```python
from build123d import *

# Parameters (mm, degrees)
SKETCH1_R                  = 2.25
BOSS_EXTRUDE1_DEPTH        = 5
M3_5_CLEARANCE_HOLE1_D     = 3.9
M3_5_CLEARANCE_HOLE1_DEPTH = 10
M3_5_CLEARANCE_HOLE1_TIP   = 1.171678207
EXTRUDE_START              = 3
SKETCH_2_R                 = 5
SKETCH_2_R_2               = 1.95
EXTRUDE_2_DEPTH            = 3


with BuildPart() as part:
    # Sketch1 → Boss-Extrude1 (new body)
    with BuildSketch(Plane.XY):
        with BuildLine():
            Line((41.849999868, 40.621529794), (20.610605728, 84.460506241))
            ThreePointArc((20.610605728, 84.460506241), (18.105708126, 87.253517924), (14.499999983, 88.289999977))
            Line((14.499999983, 88.289999977), (-24.945583467, 79.961565754))
            ThreePointArc((-24.945583467, 79.961565754), (-40.125494586, 68.851065128), (-41.843761596, 50.118193373))
            Line((-41.843761596, 50.118193373), (-27.999999977, 9.999999991))
            Line((-27.999999977, 9.999999991), (-22.999999995, 9.999999991))
            Line((-22.999999995, 9.999999991), (-22.999999995, 3.999999991))
            Line((-22.999999995, 3.999999991), (22.999999995, 3.999999991))
            Line((22.999999995, 3.999999991), (22.999999995, 9.999999991))
            Line((22.999999995, 9.999999991), (27.999999977, 9.999999991))
            Line((27.999999977, 9.999999991), (41.849999868, 21.621529803))
            Line((41.849999868, 21.621529803), (41.849999868, 40.621529794))
        make_face()
        with Locations((-29.082392063, 69.767309235)):
            Circle(SKETCH1_R, mode=Mode.SUBTRACT)
        with Locations((-34.70344114, 61.739619201)):
            Circle(SKETCH1_R, mode=Mode.SUBTRACT)
        with Locations(Location((5.43500903, 33.63437382, 0), (0, 0, 180))):
            Circle(SKETCH1_R, mode=Mode.SUBTRACT)
        with Locations(Location((11.056058107, 41.662063854, 0), (0, 0, 180))):
            Circle(SKETCH1_R, mode=Mode.SUBTRACT)
        Polygon((-22.70847113, 71.896424529), (-34.524145719, 55.021892416), (-0.938911903, 31.505258526), (10.876762686, 48.379790638), align=None, mode=Mode.SUBTRACT)
    extrude(amount=-BOSS_EXTRUDE1_DEPTH)

    # M3.5 Clearance Hole1
    with Locations(Plane.XY):
        with Locations((14.499999983, 81.499999989)):
            Hole(M3_5_CLEARANCE_HOLE1_D / 2, depth=M3_5_CLEARANCE_HOLE1_DEPTH)
            with Locations((0, 0, -(M3_5_CLEARANCE_HOLE1_DEPTH + M3_5_CLEARANCE_HOLE1_TIP / 2))):  # 118° drill point
                Cone(0, M3_5_CLEARANCE_HOLE1_D / 2, M3_5_CLEARANCE_HOLE1_TIP, mode=Mode.SUBTRACT)

    # 草图2 → 凸台-拉伸2 (add)
    with BuildSketch(Plane(origin=(0, 0, -5), x_dir=(-1, 0, 0), z_dir=(0, 0, -1)).offset(EXTRUDE_START)):
        with Locations(Location((-14.499999983, 81.499999989, 0), (0, 0, 180))):
            Circle(SKETCH_2_R)
        with Locations(Location((-14.499999983, 81.499999989, 0), (0, 0, 180))):
            Circle(SKETCH_2_R_2, mode=Mode.SUBTRACT)
    extrude(amount=-EXTRUDE_2_DEPTH)


solid = part.part
```
The model under review builds one solid part; all positions refer to its coordinate system, in mm. A direction names the side the tool comes from. Round coordinates to 2 decimals unless told otherwise and drop trailing zeros. Loops run counter-clockwise (first coordinate to the right, second up) from the corner with the lowest first, then second, coordinate; pieces in that order, holes last.
1) Wall thickness on line 1 along Y through (x, z) = (14.5, -7.1); line 2 along X through (y, z) = (40.5, -2.75); line 3 along Z through (x, y) = (10.5, 64.5): over which ranges is each line inside the solid? List them lowest first.
Values follow:
line 1: y = 76.5 to 79.55, 83.45 to 86.5
line 2: x = -38.52 to -13.78, 5.36 to 9.13, 12.98 to 41.85
line 3: z = -5 to 0
2) The part is to be moulded in two halves that separate along Y. For faces 1 (the face through (34.83, 15.73, -2.46)), 2 (the face through (-17.97, 43.43, -2.46)), 3 (the face through (31.38, 62.23, -2.46)), 4 (the face through (12.84, 43.03, -2.46)), say which applies: pulls with the +Y half, pulls with the -Y half, needs draft (parallel to the pull), parting line crosses it, or undercut.
Values follow:
face 1: pulls with the -Y half
face 2: undercut
face 3: pulls with the +Y half
face 4: undercut
3) Consider section A-A on y = 81.5. State the section outline as (x, z) points.
Values follow:
outline: (-17.66, -5) - (9.5, -5) - (9.5, -8) - (12.55, -8) - (12.55, 0) - (-17.66, 0) - close; (16.45, -8) - (19.5, -8) - (19.5, -5) - (22.04, -5) - (22.04, 0) - (16.45, 0) - close
4) Consider section B-B on x = -21. State the section outline as (y, z) points.
Values follow:
outline: (4, -5) - (45.55, -5) - (45.55, 0) - (4, 0) - close; (70.7, -5) - (80.79, -5) - (80.79, 0) - (70.7, 0) - close
5) Clearance check with flat-ended pins moving along their axes: P1, Ø2.5, axis at x = 14.5, y = 81.5, coming from the -Z side; P2, Ø1.5, axis at y = 72, z = -2.5, coming from the -X side; P3, Ø4, axis at x = -25.5, z = -2.5, coming from the -Y side; P4, Ø4, axis at x = 6.5, z = -2, coming from the +Y side. State where each tip first meets the part, or that it passes through.
Values follow:
P1: passes through
P2: stops at x = -38.56
P3: stops at y = 10
P4: stops at y = 87.02
6) Consider section D-D on x = -7.5. State the section outline as (y, z) points, then the cut area to 3 significant figures.
Values follow:
outline: (4, -5) - (36.1, -5) - (36.1, 0) - (4, 0) - close; (61.25, -5) - (83.64, -5) - (83.64, 0) - (61.25, 0) - close
area: 272 mm2
7) Consider section C-C on z = -2.5. Give the number of separate pieces and of enclosed holes in the cut face, then the cut area to 3 significant figures.
Values follow:
separate pieces: 1
enclosed holes: 6
area: 4,620 mm2
8) Tool access review of faces 5 (the face through (25, 10, -2)), 6 (the face through (-26, 10, -2)), 7 (the face through (4.886, 39.824, -2.465)), 8 (the face through (13.42, 86.38, -6.52)): name each direction out of +Z, -Z, +X, -X, +Y, -Y from which nothing blocks a thin tool from reaching the whole face with its end or side.
Values follow:
face 5: +Z, -Z, +X, -Y
face 6: +Z, -Z, -X, -Y
face 7: +Z, -Z
face 8: -Z
